CAD build for the part. Positions are in the model's coordinates, mm. A direction names the side the tool comes from. Coordinates: 2 decimals unless noted, no trailing zeros. Order: outer loops, then holes, each group sorted by start corner. A loop starts at its lowest first (then second) coordinate and runs counter-clockwise, first axis right, second up. Notation, with made-up numbers: (79, 19) - (109, 19) arc R9 cw to (109, 26) - close; hole circle Ø9 at (31, 11). An arc over 180 degrees is marked (long way). Return JSON: item names as keys, results as strings.
from build123d import *

# Parameters (mm, degrees)
SKETCH1_R           = 4.5
BOSS_EXTRUDE1_DEPTH = 5
CIRPATTERN1_COUNT   = 12


with BuildPart() as part:
    # Sketch1 → Boss-Extrude1 (new body, symmetric)
    with BuildSketch(Plane.XY):
        with BuildLine():
            Line((-1, 6.916079783), (-1, 5.916079783))
            ThreePointArc((-1, 5.916079783), (0, -6), (1, 5.916079783))
            Line((1, 5.916079783), (1, 6.916079783))
            Line((1, 6.916079783), (0.5, 8.116079783))
            Line((0.5, 8.116079783), (-0.5, 8.116079783))
            Line((-0.5, 8.116079783), (-1, 6.916079783))
        make_face()
        Circle(SKETCH1_R, mode=Mode.SUBTRACT)
    boss_extrude1 = extrude(amount=BOSS_EXTRUDE1_DEPTH, both=True)

    # CirPattern1: Boss-Extrude1 ×12 about axis
    cirpattern1_axis = Axis((0, 0, 0), (0, 0, 1))
    for i in range(1, CIRPATTERN1_COUNT):
        add(boss_extrude1.rotate(cirpattern1_axis, i * 360 / CIRPATTERN1_COUNT))


solid = part.part
Item 1: Which spindle directions (+Z, -Z, +X, -X, +Y, -Y) get a long thin tool onto all of the face, cutting with end or side? Do faces 1 (the flat face through (5.1, 4.1, 0.1)), 2 (the flat face through (5.1, -4.1, 0.1)), 3 (the flat face through (7.025, -4.064, 0.07)), 4 (the flat face through (4.41, -6.14, 0.07)), 5 (the flat face through (-6.4, 1, 0.1)). Say none if no direction does.
Findings below:
{"face 1": "+Z, -Z, +Y", "face 2": "+Z, -Z, -Y", "face 3": "+Z, -Z, +X, -Y", "face 4": "+Z, -Z, +X", "face 5": "+Z, -Z, -X"}
Item 2: Drop flat-ended pins along their axis: P1, Ø1.1, axis at x = -6.5, z = 1.5, coming from the -Y side; P2, Ø0.8, axis at x = -6, z = -1, coming from the +Y side; P3, Ø3, axis at x = 5, z = -2, coming from the -Y side; P4, Ø5.5, axis at x = 0, y = 0, coming from the +Z side. Give the stop position or say it passes through.
Findings below:
{"P1": "stops at y = -4.49", "P2": "stops at y = 4.44", "P3": "stops at y = -7.28", "P4": "passes through"}
Item 3: Band-saw the part on A-A, the plane x = 0. List the corners of the cut face in (y, z), then the cut area to 3 significant figures.
Findings below:
{"outline": "(-8.12, -5) - (-4.5, -5) - (-4.5, 5) - (-8.12, 5) - close; (4.5, -5) - (8.12, -5) - (8.12, 5) - (4.5, 5) - close", "area": "72.3 mm²"}
Item 4: Wall check: L1, parallel to X at y = 0, z = 1.75; L2, parallel to Y at x = 7, z = -2. Give the ranges that are in metal, low to high. Write a range as [from, to].
Findings below:
{"L1": "x = [-8.12, -4.5], [4.5, 8.12]", "L2": "y = [-4.11, -3.26], [-0.97, 0.97], [3.26, 4.11]"}
Item 5: Mould opens along X. For faces 6 (the flat face through (6.4, 1, 0.1)), 7 (the cylindrical face through (-5.793, 1.561, 0.07)), 8 (the flat face through (-6.125, 4.406, 0.07)) say: released by +X, released by -X, zero draft, split by the parting line, or undercut.
Findings below:
{"face 6": "zero draft", "face 7": "released by -X", "face 8": "undercut"}
Item 6: Band-saw the part on C-C, the plane y = -5. List the corners of the cut face in (x, z), then the cut area to 3 significant figures.
Findings below:
{"outline": "(-4.04, -5) - (4.04, -5) - (4.04, 5) - (-4.04, 5) - close", "area": "80.8 mm²"}
